Geometry check sheet. Reference: the model listing, model coordinates, mm. A direction names the side the tool comes from. Give positions to 0.01 mm unless a question says otherwise; leave off trailing zeros. Loops run counter-clockwise (first coordinate to the right, second up) from the corner with the lowest first, then second, coordinate; pieces in that order, holes last. Notation, with made-up numbers: (77.5, 61) - (94.5, 61) arc R25 cw to (94.5, 90) - close; hole circle Ø9 at (66.25, 61.5). An arc over 180 degrees is marked (long way). Use a Markdown table: item, result. Add a question column.
1. Draft check along Y on faces 1 (the conical face through (91.87, 0.1, -25.43)), 2 (the cylindrical face through (105.378, -10.618, 13.848)), 3 (the cylindrical face through (98.194, 0.329, -22.494)), 4 (the flat face through (153.924, 0, 0)). Enter one of: pulls with the +Y half, pulls with the -Y half, needs draft (parallel to the pull), parting line crosses it, or undercut.
2. Cross-section at A-A on x = 95. Enter the section's corners in (y, z).
3. Depth check by flat-ended pin: P1, Ø6, axis at x = 50.5, y = 25, coming from the +Z side; P2, Ø1.5, axis at x = 43, y = -3.5, coming from the -Z side; P3, Ø10, axis at x = 60.5, y = 21.5, coming from the -Z side; P4, Ø6.5, axis at y = -25, z = 0, coming from the -X side. Enter the tip coordinate at first touch or a pass-through.
4. Cross-section at D-D on x = 46. Enter the section's corners in (y, z), and give its area (3 significant figures).
5. Set-up check for faces 5 (the cylindrical face through (50.84, -23.96, 31.24)), 6 (the flat face through (107.696, 0, -8)): record each of +Z, -Z, +X, -X, +Y, -Y from which the full face is reachable in a straight line by a thin tool's end or side.
6. Cross-section at C-C on z = 20.5. Enter the section's corners in (x, y).
7. Cross-section at B-B on y = 9. Enter the section's corners in (x, z).
8. Material ranges on L1, parallel to Y at x = 98.25, z = 0; L2, parallel to X at y = 6, z = -6.5; L3, parallel to X at y = -19, z = 32, recorded low to high.
from build123d import *

# Parameters (mm, degrees)
SKETCH1_R           = 39.37
BOSS_EXTRUDE1_DEPTH = 103.124
BOSS_EXTRUDE2_DEPTH = 50.8
CIRPATTERN1_COUNT   = 4
SKETCH6_R           = 17.4498
SKETCH6_R_2         = 6.35
BOSS_EXTRUDE3_DEPTH = 4.572


with BuildPart() as part:
    # Sketch1 → Boss-Extrude1 (new body)
    with BuildSketch(Plane(origin=(0, 0, 0), x_dir=(0, 0, -1), z_dir=(1, 0, 0))):
        Circle(SKETCH1_R)
    extrude(amount=BOSS_EXTRUDE1_DEPTH)

    # Sketch2 → Boss-Extrude2 (add)
    with BuildSketch(Plane(origin=(103.124, 0, 0), x_dir=(0, 0, -1), z_dir=(1, 0, 0))):
        with BuildLine():
            Line((-1.5875, 6.148361062), (-1.5875, 4.560861062))
            Line((-1.5875, 4.560861062), (1.5875, 4.560861062))
            Line((1.5875, 4.560861062), (1.5875, 6.148361062))
            ThreePointArc((1.5875, 6.148361062), (0, -6.35), (-1.5875, 6.148361062))
        make_face()
    extrude(amount=BOSS_EXTRUDE2_DEPTH)

    # Sketch4 → #8 (0.199) Diameter Hole1 (revolve, cut)
    with BuildSketch(Plane(origin=(103.124, 25, 0), x_dir=(0, 0, -1), z_dir=(0, 1, 0))):
        Polygon((0, 0), (0, 11.518555042), (2.5273, 10), (2.5273, 0), align=None)
    f_8_0_199_diameter_hole1 = revolve(axis=Axis((109.474, 25, 0), (-1, 0, 0)), mode=Mode.SUBTRACT)

    # CirPattern1: #8 (0.199) Diameter Hole1 ×4 about axis
    cirpattern1_axis = Axis((0, 0, 0), (1, 0, 0))
    for i in range(1, CIRPATTERN1_COUNT):
        add(f_8_0_199_diameter_hole1.rotate(cirpattern1_axis, i * 360 / CIRPATTERN1_COUNT), mode=Mode.SUBTRACT)

    # Sketch6 → Boss-Extrude3 (add)
    with BuildSketch(Plane(origin=(103.124, 0, 0), x_dir=(0, 0, -1), z_dir=(1, 0, 0))):
        Circle(SKETCH6_R)
        Circle(SKETCH6_R_2, mode=Mode.SUBTRACT)
    extrude(amount=BOSS_EXTRUDE3_DEPTH)


solid = part.part
Values found:
| question | item | result |
|---|---|---|
| 1 | face 1 | undercut |
| 1 | face 2 | parting line crosses it |
| 1 | face 3 | undercut |
| 1 | face 4 | needs draft |
| 2 | outline | circle Ø78.74 at (0, 0); hole circle Ø5.05 at (-25, 0); hole circle Ø5.05 at (0, -25); hole circle Ø5.05 at (0, 25); hole circle Ø5.05 at (25, 0) |
| 3 | P1 | stops at z = 32.65 |
| 3 | P2 | stops at z = -39.27 |
| 3 | P3 | stops at z = -35.75 |
| 3 | P4 | stops at x = 0 |
| 4 | outline | circle Ø78.74 at (0, 0) |
| 4 | area | 4,870 mm2 |
| 5 | face 5 | +X, -X |
| 5 | face 6 | +X |
| 6 | outline | (0, -33.61) - (103.12, -33.61) - (103.12, 33.61) - (0, 33.61) - close |
| 7 | outline | (0, -38.33) - (103.12, -38.33) - (103.12, -14.95) - (107.7, -14.95) - (107.7, 14.95) - (103.12, 14.95) - (103.12, 38.33) - (0, 38.33) - close |
| 8 | L1 | y = -39.37 to -27.53, -22.47 to 22.47, 27.53 to 39.37 |
| 8 | L2 | x = 0 to 107.7 |
| 8 | L3 | x = 0 to 103.12 |
